Part model, mm, in its own coordinate system. A direction names the side the tool comes from. Round coordinates to 2 decimals unless told otherwise and drop trailing zeros. Write each loop counter-clockwise with the first axis right and the second up, starting at its lowest first coordinate (ties: lowest second). Pieces come first, ordered by that corner, then holes. Notation, with made-up numbers: (5.5, -25.75) -> (9.5, -25.75) arc R33 ccw to (9.5, 3.25) -> close; hole circle Ø3 at (-12.75, -19.75). An arc over 180 degrees is marked (long way). Use CSV: the item, a comma, the result in double quotes. Start each with the question number.
```python
from build123d import *

# Parameters (mm, degrees)
BOSS_EXTRUDE1_DEPTH = 5
SKETCH2_W           = 12
SKETCH2_H           = 26
CUT_EXTRUDE1_DEPTH  = 6
SKETCH3_R           = 1.25
CUT_EXTRUDE2_DEPTH  = 6
SKETCH4_R           = 1.23
CUT_EXTRUDE3_DEPTH  = 13
SKETCH5_W           = 98
SKETCH5_H           = 10
CUT_EXTRUDE4_DEPTH  = 3
SKETCH6_W           = 98
SKETCH6_H           = 6
CUT_EXTRUDE5_DEPTH  = 1
CHAMFER1_SIZE       = 1


with BuildPart() as part:
    # Sketch1 → Boss-Extrude1 (new body)
    with BuildSketch(Plane.XY):
        Polygon((-61, 17.8), (-59.8, 19), (59.8, 19), (61, 17.8), (61, -19), (-61, -19), align=None)
    extrude(amount=BOSS_EXTRUDE1_DEPTH)

    # Sketch2 → Cut-Extrude1 (cut, through all)
    with BuildSketch(Plane.XY.offset(5)):
        with Locations((55, -6)):
            Rectangle(SKETCH2_W, SKETCH2_H)
    cut_extrude1 = extrude(amount=-CUT_EXTRUDE1_DEPTH, mode=Mode.SUBTRACT)

    # Sketch3 → Cut-Extrude2 (cut, through all)
    with BuildSketch(Plane.XY.offset(5)):
        with Locations((42, 9)):
            Circle(SKETCH3_R)
        with Locations((42, 3.5)):
            Circle(SKETCH3_R)
        with Locations((-38, 9)):
            Circle(SKETCH3_R)
        with Locations((-38, 3.5)):
            Circle(SKETCH3_R)
    extrude(amount=-CUT_EXTRUDE2_DEPTH, mode=Mode.SUBTRACT)

    # Sketch4 → Cut-Extrude3 (cut, through all)
    with BuildSketch(Plane.XZ.offset(-7)):
        with Locations((56, 2.5)):
            Circle(SKETCH4_R)
    cut_extrude3 = extrude(amount=-CUT_EXTRUDE3_DEPTH, mode=Mode.SUBTRACT)

    # Mirror1: Cut-Extrude1, Cut-Extrude3 across plane
    add(cut_extrude1.mirror(Plane(origin=(0, 0, 0), x_dir=(0, 0, 1), z_dir=(1, 0, 0))), mode=Mode.SUBTRACT)
    add(cut_extrude3.mirror(Plane(origin=(0, 0, 0), x_dir=(0, 0, 1), z_dir=(1, 0, 0))), mode=Mode.SUBTRACT)

    # Sketch5 → Cut-Extrude4 (cut)
    with BuildSketch(Plane.XY.offset(5)):
        with Locations((0, -14)):
            Rectangle(SKETCH5_W, SKETCH5_H)
    extrude(amount=-CUT_EXTRUDE4_DEPTH, mode=Mode.SUBTRACT)

    # Sketch6 → Cut-Extrude5 (cut)
    with BuildSketch(Plane(origin=(0, 0, 0), x_dir=(-1, 0, 0), z_dir=(0, 0, -1))):
        with Locations((0, -16)):
            Rectangle(SKETCH6_W, SKETCH6_H)
    extrude(amount=-CUT_EXTRUDE5_DEPTH, mode=Mode.SUBTRACT)

    # Chamfer1
    chamfer1_edges = [part.edges().sort_by_distance(p)[0] for p in [
        (0, -9, 5),
    ]]
    chamfer(chamfer1_edges, length=CHAMFER1_SIZE)


solid = part.part
```
1. Band-saw the part on B-B (x = 56). List the corners of the cut face in (y, z), then the cut area to 3 significant figures.
2. Drill centre lines: line 1 along Y through (x, z) = (-38, 1.2); line 2 along Y through (x, z) = (-38, 2.35); line 3 along Z through (x, y) = (56, 15.5). Where is each one in solid material? Low to high. Write a range as [from, to].
3. Which spindle directions (+Z, -Z, +X, -X, +Y, -Y) get a long thin tool onto all of the face, cutting with end or side? Do faces 4 (the flat face through (49, -3, 3)), 5 (the flat face through (-1, -14, 2)), 6 (the flat face through (1, -16, 1)). Say none if no direction does.
4. Pull direction X, two halves, no side cores. Call faces 1 (the flat face through (61, 12, 2)), 2 (the cylindrical face through (-54.77, 12.92, 2.55)), 3 (the flat face through (-1, 19, 2)): released by +X, released by -X, zero draft, split by the parting line, or undercut.
5. Flat gauge pins, fed straight in: pin 1 (1.8 mm diameter, centred on x = -3.5, y = -15, fed in from -Z); pin 2 (0.8 mm diameter, centred on x = 19, z = 0.5, fed in from -Y); pin 3 (3 mm diameter, centred on x = 46, y = -14.5, fed in from +Z); pin 4 (3 mm diameter, centred on x = -3, y = 14, fed in from -Z). Where does each tip first touch, or does it go through?
6. Band-saw the part on A-A (y = 9). List the corners of the cut face in (x, z), then the cut area to 3 significant figures.
7. Band-saw the part on D-D (x = 30). List the corners of the cut face in (y, z).
8. Band-saw the part on C-C (x = -38). List the corners of the cut face in (y, z), then the cut area to 4 significant figures.
Answers below:
1,outline,"(7, 0) -> (19, 0) -> (19, 1.27) -> (7, 1.27) -> close; (7, 3.73) -> (19, 3.73) -> (19, 5) -> (7, 5) -> close"
1,area,"30.5 mm^2"
2,line 1,"y = [-19, 2.25], [4.75, 7.75], [10.25, 19]"
2,line 2,"y = [-9, 2.25], [4.75, 7.75], [10.25, 19]"
2,line 3,"z = [0, 1.27], [3.73, 5]"
3,face 4,"+Z, -Z, +X, -Y"
3,face 5,"+Z, +X, -X, -Y"
3,face 6,"-Z, +X, -X, -Y"
4,face 1,"released by +X"
4,face 2,"undercut"
4,face 3,"zero draft"
5,pin 1,"stops at z = 1"
5,pin 2,"stops at y = -13"
5,pin 3,"stops at z = 2"
5,pin 4,"stops at z = 0"
6,outline,"(-61, 0) -> (-39.25, 0) -> (-39.25, 5) -> (-61, 5) -> close; (-36.75, 0) -> (40.75, 0) -> (40.75, 5) -> (-36.75, 5) -> close; (43.25, 0) -> (61, 0) -> (61, 5) -> (43.25, 5) -> close; hole circle Ø2.46 at (-56, 2.5); hole circle Ø2.46 at (56, 2.5)"
6,area,"575 mm^2"
7,outline,"(-19, 1) -> (-13, 1) -> (-13, 0) -> (19, 0) -> (19, 5) -> (-8, 5) -> (-9, 4) -> (-9, 2) -> (-19, 2) -> close"
8,outline,"(-19, 1) -> (-13, 1) -> (-13, 0) -> (2.25, 0) -> (2.25, 5) -> (-8, 5) -> (-9, 4) -> (-9, 2) -> (-19, 2) -> close; (4.75, 0) -> (7.75, 0) -> (7.75, 5) -> (4.75, 5) -> close; (10.25, 0) -> (19, 0) -> (19, 5) -> (10.25, 5) -> close"
8,area,"128.5 mm^2"
